Source: CAD feature listing. Evaluate the final solid. Frame: model axes, mm. A direction names the side the tool comes from. Round coordinates to 2 decimals unless told otherwise and drop trailing zeros. Loops run counter-clockwise (first coordinate to the right, second up) from the corner with the lowest first, then second, coordinate; pieces in that order, holes last. Notation, with made-up numbers: (45, 86) - (52, 86) arc R26 cw to (52, 104) - close; hole circle Ø4 at (-2.75, 43). An arc over 180 degrees is marked (long way). One line per question, with ' | ' between items. Start each with the question number.
1. Ray query, line 1 (X direction, y = 22.25, z = 9); line 2 (Z direction, x = 0, y = 17.25); line 3 (Y direction, x = 6.75, z = 9). Return the intervals inside material, ascending.
2. Cut plane B-B (x = 10.25). Return loops of the section in (y, z).
3. Cut plane D-D (z = 3.5). Return loops of the section in (x, y).
4. Access query for faces 1 (the flat face through (-14, 5, 9)), 2 (the cylindrical face through (0, 15, 7)). Directions: +Z, -Z, +X, -X, +Y, -Y. A direction counts if a zero-diameter tool reaches every point of the face in a straight line with its end or side. Return the directions, or none.
5. Mould query, pull axis Y, two halves, no side actions, for faces 3 (the cylindrical face through (4.87, -9.1, 11.86)), 4 (the flat face through (-4, -10, 9)), 5 (the flat face through (0, 0, 18)), 6 (the flat face through (5, -30, 9)). Classes: pulls with the +Y half, pulls with the -Y half, needs draft (parallel to the pull), parting line crosses it, or undercut.
6. Cut plane C-C (y = -10). Return loops of the section in (x, z), then the cut area to 3 significant figures.
7. Pin query (flat end, axial travel): pin 1 (2 mm diameter, centred on x = -11, z = 3, fed in from -Y). Return the tip coordinate at first contact, or that it passes through.
8. Cut plane A-A (y = 19). Return loops of the section in (x, z), then the cut area to 3 significant figures.
```python
from build123d import *

# Parameters (mm, degrees)
SKETCH1_W                    = 28
SKETCH1_H                    = 60
BOSS_EXTRUDE1_DEPTH          = 18
CHAMFER1_SIZE                = 10
F_4_0_4_DIAMETER_HOLE1_D     = 4
F_4_0_4_DIAMETER_HOLE1_DEPTH = 30
F_4_0_4_DIAMETER_HOLE1_TIP   = 1.201721238
F_6_0_6_DIAMETER_HOLE2_D     = 6
F_6_0_6_DIAMETER_HOLE2_DEPTH = 18


with BuildPart() as part:
    # Sketch1 → Boss-Extrude1 (new body)
    with BuildSketch(Plane.XY):
        Rectangle(SKETCH1_W, SKETCH1_H)
    extrude(amount=BOSS_EXTRUDE1_DEPTH)

    # Chamfer1
    chamfer1_edges = [part.edges().sort_by_distance(p)[0] for p in [
        (-14, -30, 9),
    ]]
    chamfer(chamfer1_edges, length=CHAMFER1_SIZE)

    # Ø4.0 (4) Diameter Hole1
    with Locations(Plane(origin=(0, 30, 0), x_dir=(1, 0, 0), z_dir=(0, 1, 0))):
        with Locations((0, -9)):
            Hole(F_4_0_4_DIAMETER_HOLE1_D / 2, depth=F_4_0_4_DIAMETER_HOLE1_DEPTH)
            with Locations((0, 0, -(F_4_0_4_DIAMETER_HOLE1_DEPTH + F_4_0_4_DIAMETER_HOLE1_TIP / 2))):  # 118° drill point
                Cone(0, F_4_0_4_DIAMETER_HOLE1_D / 2, F_4_0_4_DIAMETER_HOLE1_TIP, mode=Mode.SUBTRACT)

    # Ø6.0 (6) Diameter Hole2
    with Locations(Plane(origin=(14, 0, 0), x_dir=(0, 0, -1), z_dir=(1, 0, 0))):
        with Locations((-9, -10)):
            Hole(F_6_0_6_DIAMETER_HOLE2_D / 2, depth=F_6_0_6_DIAMETER_HOLE2_DEPTH)


solid = part.part
```
Answers follow:
1) line 1: x = -14 to -2, 2 to 14 | line 2: z = 0 to 7, 11 to 18 | line 3: y = -30 to -13, -7 to 30
2) outline: (-30, 0) - (30, 0) - (30, 18) - (-30, 18) - close; hole circle Ø6 at (-10, 9)
3) outline: (-14, -20) - (-4, -30) - (14, -30) - (14, 30) - (-14, 30) - close
4) face 1: +Z, -Z, -X, +Y, -Y | face 2: +Y
5) face 3: undercut | face 4: undercut | face 5: needs draft | face 6: pulls with the -Y half
6) outline: (-14, 0) - (14, 0) - (14, 6) - (-4, 6) - (-4, 12) - (14, 12) - (14, 18) - (-14, 18) - close | area: 396 mm2
7) pin 1: stops at y = -24
8) outline: (-14, 0) - (14, 0) - (14, 18) - (-14, 18) - close; hole circle Ø4 at (0, 9) | area: 491 mm2
